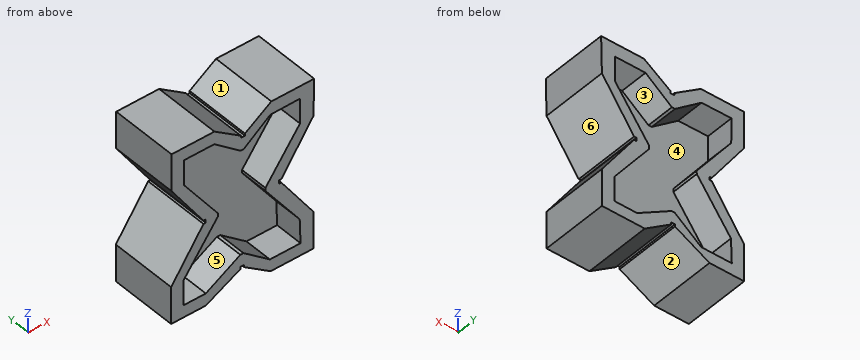
```python
from build123d import *

# Parameters (mm, degrees)
F1_DEPTH = 90.1446
F4_DEPTH = 38.1
F7_DEPTH = 38.1


with BuildPart() as f1:
    # F0 (on Front) → F1 (new body)
    with BuildSketch(Plane.XZ):
        Polygon((-11.1971926081, 65.7086565368), (-69.1091926081, 65.7086565368), (-69.1091926081, 15.8992565368), (-26.0065842281, -46.8154278155), (-22.9906474179, -46.8154278155), (-22.9906474179, -51.3447030535), (-26.0065842281, -51.3447030535), (-69.729202812, -113.6287227273), (-69.729202812, -163.4422105699), (-22.8745764246, -163.4422105699), (23.7734285709, -138.940374625), (23.7734285709, -135.9147534492), (28.9550285709, -135.9147534492), (28.9550285709, -138.9272423858), (64.6245286164, -163.4422105699), (122.5365286164, -163.4422105699), (122.5365286164, -113.6328105699), (79.1036308243, -51.1464130746), (76.0683308243, -51.1464130746), (76.0683308243, -46.5761250044), (79.1036308243, -46.5761250044), (122.5365286164, 15.9102724908), (123.5840374592, 65.7086565368), (65.6720374592, 65.7086565368), (30.0025374137, 41.1936883527), (30.0025374137, 38.175295005), (24.4723074374, 38.175295005), (24.4723074374, 41.1936883527), align=None)
    extrude(amount=-F1_DEPTH)

    # F3 (on offset) → F4 (cut)
    with BuildSketch(Plane.XZ):
        Polygon((-6.4795594404, -51.5769487249), (-53.295402812, -113.7468837801), (-53.295402812, -146.9806581736), (-22.8745764246, -147.0209074169), (23.7734285709, -119.4822192192), (28.0406285709, -119.4822192192), (63.7101286164, -146.9806581736), (105.0975570712, -146.9717806065), (103.9679117275, -113.9575218417), (57.8230765612, -51.2830203653), (57.6468469615, -47.0311700371), (104.3438033673, 15.2281126267), (104.5963698348, 48.9120816117), (64.1748463129, 48.43781649), (28.3937643672, 21.0621996767), (24.126596129, 21.0786637873), (-11.4306816807, 48.7568000231), (-52.5953805913, 48.7568000231), (-52.5953805913, 15.3812000231), (-6.4795594404, -47.3097487249), align=None)
    extrude(amount=-F4_DEPTH, mode=Mode.SUBTRACT)

    # F6 (on offset) → F7 (cut)
    with BuildSketch(Plane(origin=(0, 90.1446, 0), x_dir=(-1, 0, 0), z_dir=(0, 1, 0))):
        Polygon((-58.6403822024, -52.5351678955), (-105.456225574, -114.7051029507), (-105.456225574, -147.9388773441), (-75.0353991867, -147.9791265874), (-28.3873941911, -120.4404383898), (-24.1201941911, -120.4404383898), (11.5493058543, -147.9388773441), (52.9367343092, -147.9299997771), (51.8070889654, -114.9157410123), (5.6622537992, -52.2412395359), (5.4860241995, -47.9893892076), (52.1829806052, 14.2698934561), (52.4355470727, 47.9538624411), (12.0140235509, 47.4795973194), (-23.7670583948, 20.1039805062), (-28.034226633, 20.1204446167), (-63.5915044428, 47.7985808526), (-104.7562033534, 47.7985808526), (-104.7562033534, 14.4229808526), (-58.6403822024, -48.2679678955), align=None)
    extrude(amount=-F7_DEPTH, mode=Mode.SUBTRACT)


solid = f1.part
```
Geometry check sheet. Reference: the model listing, model coordinates, mm. Face numbers are marked on the shaded views. A direction names the side the tool comes from. Round coordinates to 2 decimals unless told otherwise and drop trailing zeros. Order: outer loops, then holes, each group sorted by start corner. A loop starts at its lowest first (then second) coordinate and runs counter-clockwise, first axis right, second up. Notation, with made-up numbers: M -31,-31.75 L -27,-31.75 A11 cw -27,-25.75 Z; hole C -5.75,-8 d9. An arc over 180 degrees is marked long. Write item = value, one per line.
Q1. Depth check by flat-ended pin: pin 1 Ø3.5 at (y, z) = (51, -48) entering from +X; pin 2 Ø2.5 at (y, z) = (52, 40) entering from -X; pin 3 Ø1 at (x, y) = (14.5, 26.5) entering from -Z. Enter the tip coordinate at first touch or a pass-through.
Answer block:
pin_1 = 79.33
pin_2 = -69.11
pin_3 = -144.07
Q2. Section check C-C (z = -36.5). Enter the section's corners in (x, y).
Answer block:
outline = M -33.1,0 L -14.43,0 L -14.43,38.1 L 65.55,38.1 L 65.55,0 L 86.11,0 L 86.11,90.14 L 67.3,90.14 L 67.3,52.04 L -14.1,52.04 L -14.1,90.14 L -33.1,90.14 Z
Q3. Section check A-A (x = 85). Enter the section's corners in (y, z), plus the area to 3 significant figures.
Answer block:
outline = M 0,-163.44 L 90.14,-163.44 L 90.14,-147.97 L 52.04,-147.97 L 52.04,-87.54 L 90.14,-87.54 L 90.14,-59.63 L 0,-59.63 L 0,-88.2 L 38.1,-88.2 L 38.1,-146.98 L 0,-146.98 Z; M 0,-38.09 L 90.14,-38.09 L 90.14,-12.43 L 52.04,-12.43 L 52.04,47.8 L 90.14,47.8 L 90.14,65.71 L 0,65.71 L 0,48.68 L 38.1,48.68 L 38.1,-10.56 L 0,-10.56 Z
area = 9,620 mm^2
Q4. Section check B-B (y = 44.5). Enter the section's corners in (x, z).
Answer block:
outline = M -69.73,-163.44 L -22.87,-163.44 L 23.77,-138.94 L 23.77,-135.91 L 28.96,-135.91 L 28.96,-138.93 L 64.62,-163.44 L 122.54,-163.44 L 122.54,-113.63 L 79.1,-51.15 L 76.07,-51.15 L 76.07,-46.58 L 79.1,-46.58 L 122.54,15.91 L 123.58,65.71 L 65.67,65.71 L 30,41.19 L 30,38.18 L 24.47,38.18 L 24.47,41.19 L -11.2,65.71 L -69.11,65.71 L -69.11,15.9 L -26.01,-46.82 L -22.99,-46.82 L -22.99,-51.34 L -26.01,-51.34 L -69.73,-113.63 Z
Q5. Release check for a two-part mould opening along Z. For the marked faces 1, 2 and 3 record: released by +Z, released by -Z, zero draft, split by the parting line, or undercut.
Answer block:
face_1 = released by +Z
face_2 = released by -Z
face_3 = undercut
Q6. Section check D-D (x = 10.5). Enter the section's corners in (y, z).
Answer block:
outline = M 0,-145.91 L 90.14,-145.91 L 90.14,-130.94 L 52.04,-130.94 L 52.04,30.25 L 90.14,30.25 L 90.14,50.8 L 0,50.8 L 0,31.69 L 38.1,31.69 L 38.1,-127.32 L 0,-127.32 Z
Q7. Set-up check for the marked faces 4, 5 and 6: record each of +Z, -Z, +X, -X, +Y, -Y from which the full face is reachable in a straight line by a thin tool's end or side.
Answer block:
face_4 = +Y
face_5 = -Y
face_6 = +X, +Y, -Y
Q8. Scan lines: line 1 (Z direction, x = -9, y = 27.5); line 2 (Z direction, x = -17.5, y = 26); line 3 (Z direction, x = -26.5, y = 34). Record each from-to range of solid material in increasing order.
Answer block:
line_1 = -156.15 to -138.83, -54.92 to -43.88, 46.86 to 64.2
line_2 = -160.62 to -143.85, -66.21 to -32.33, 48.76 to 65.71
line_3 = -163.44 to -147.02, -78.16 to -52.05, -46.1 to -20.09, 48.76 to 65.71
